Read the model definition and answer for the solid it produces. Units are mm, in the model's axes. A direction names the side the tool comes from. Coordinates: 2 decimals unless noted, no trailing zeros. Loops run counter-clockwise (first coordinate to the right, second up) from the corner with the lowest first, then second, coordinate; pieces in that order, holes last. Notation, with made-up numbers: (30, 18) - (85, 18) arc R5 cw to (85, 27) - close; hole circle Ø8 at (-9.75, -1). An arc over 180 degrees is marked (long way). Use one line per item in the form item = value. Start each with the question number.
1) A cutting plane is placed at B-B (y = 0). Give the vertices of the cut face in (x, z).
2) A cutting plane is placed at D-D (y = -41.5). Give the vertices of the cut face in (x, z), and give its area (3 significant figures).
3) Consider line 1 (X direction, y = -38, z = 11); line 2 (Y direction, x = -3, z = 69.5); line 3 (Z direction, x = 12.5, y = 15). Determine where each line is inside the solid, lowest interval first.
4) Which of the six approach directions +Z, -Z, +X, -X, +Y, -Y give full straight-line access (tool end or side, diameter ignored) to faces 1 (the face through (-16.31, -19.16, 17.93)), 2 (the face through (40.94, -29.63, 35.74)), 3 (the face through (8.89, 17, 10)), 4 (the face through (-36, -92, 11)), 5 (the face through (-1, -76.2, -46))?
5) The mould has two halves that part along Z. Classify faces 6 (the face through (37, -92, 8)), 7 (the face through (-36.437, -62.42, 9.311)), 8 (the face through (-48.89, 23.59, 10.2)), 9 (the face through (-0.4, -63.3, 32.5)): released by +Z, released by -Z, zero draft, split by the parting line, or undercut.
6) Each of these flat-tipped pins is pushed along its axis until it touches: P1, Ø4, axis at x = -15.5, y = -15.5, coming from the -Z side; P2, Ø4, axis at x = -35, y = -21, coming from the +Z side; P3, Ø1, axis at x = 7, z = 1, coming from the +Y side; P4, Ø12, axis at x = -6.5, z = 9, coming from the +Y side. Where does it stop, or does it pass through?
7) A cutting plane is placed at A-A (x = 0). Give the vertices of the cut face in (y, z).
8) A cutting plane is placed at C-C (z = 10). State how many separate pieces and enclosed holes the cut face has, and give its area (3 significant figures).
from build123d import *

# Parameters (mm, degrees)
BOSS_EXTRUDE1_DEPTH = 20
SKETCH2_R           = 16.25
SKETCH2_R_2         = 2.15
CUT_EXTRUDE1_DEPTH  = 20
SKETCH5_R           = 3.75
CUT_EXTRUDE4_DEPTH  = 4.2
FILLET3_R           = 4
SKETCH6_W           = 101.6
SKETCH6_H           = 152.4
BOSS_EXTRUDE2_DEPTH = 20
SKETCH7_R           = 3.75
CUT_EXTRUDE5_DEPTH  = 4.2
SKETCH8_R           = 1.8
CUT_EXTRUDE6_DEPTH  = 60
CHAMFER1_SIZE       = 25.4
BOSS_EXTRUDE4_DEPTH = 20
FILLET4_R           = 6.35
CUT_EXTRUDE8_DEPTH  = 165.339404891
CUT_EXTRUDE9_DEPTH  = 165.339404891


with BuildPart() as part:
    # Sketch1 → Boss-Extrude1 (new body)
    with BuildSketch(Plane.XY):
        Polygon((50.8, 25.4), (8.89, 25.4), (8.89, 13.302928249), (-8.89, 13.302928249), (-8.89, 25.4), (-50.8, 25.4), (-50.8, -76.2), (50.8, -76.2), align=None)
    extrude(amount=BOSS_EXTRUDE1_DEPTH)

    # Sketch2 → Cut-Extrude1 (cut)
    with BuildSketch(Plane.XY.offset(20)):
        Circle(SKETCH2_R)
        with Locations((-15.5, -15.5)):
            Circle(SKETCH2_R_2)
        with Locations((-15.5, 15.5)):
            Circle(SKETCH2_R_2)
        with Locations((15.5, -15.5)):
            Circle(SKETCH2_R_2)
        with Locations((15.5, 15.5)):
            Circle(SKETCH2_R_2)
    extrude(amount=-CUT_EXTRUDE1_DEPTH, mode=Mode.SUBTRACT)

    # Sketch5 → Cut-Extrude4 (cut)
    with BuildSketch(Plane.XY.offset(20)):
        with Locations((-15.5, 15.5)):
            Circle(SKETCH5_R)
        with Locations((15.5, 15.5)):
            Circle(SKETCH5_R)
        with Locations((15.5, -15.5)):
            Circle(SKETCH5_R)
        with Locations((-15.5, -15.5)):
            Circle(SKETCH5_R)
    extrude(amount=-CUT_EXTRUDE4_DEPTH, mode=Mode.SUBTRACT)

    # Fillet3
    fillet3_edges = [part.edges().sort_by_distance(p)[0] for p in [
        (8.89, 13.602587989, 10),
        (-8.89, 13.602587989, 10),
    ]]
    fillet(fillet3_edges, radius=FILLET3_R)

    # Sketch6 → Boss-Extrude2 (add)
    with BuildSketch(Plane.XZ.offset(76.2)):
        with Locations((0, 10)):
            Rectangle(SKETCH6_W, SKETCH6_H)
    extrude(amount=BOSS_EXTRUDE2_DEPTH)

    # Sketch7 → Cut-Extrude5 (cut)
    with BuildSketch(Plane.XZ.offset(96.2)):
        with Locations((-38.1, 10)):
            Circle(SKETCH7_R)
        with Locations((38.1, 10)):
            Circle(SKETCH7_R)
        with Locations((0, 10)):
            Circle(SKETCH7_R)
    extrude(amount=-CUT_EXTRUDE5_DEPTH, mode=Mode.SUBTRACT)

    # Sketch8 → Cut-Extrude6 (cut)
    with BuildSketch(Plane.XZ.offset(92)):
        with Locations((-38.1, 10)):
            Circle(SKETCH8_R)
        with Locations((38.1, 10)):
            Circle(SKETCH8_R)
        with Locations((0, 10)):
            Circle(SKETCH8_R)
    extrude(amount=-CUT_EXTRUDE6_DEPTH, mode=Mode.SUBTRACT)

    # Chamfer1
    chamfer1_edges = [part.edges().sort_by_distance(p)[0] for p in [
        (0, -76.2, 0),
        (0, -76.2, 20),
    ]]
    chamfer(chamfer1_edges, length=CHAMFER1_SIZE)

    # Sketch12 → Boss-Extrude4 (add)
    with BuildSketch(Plane(origin=(50.8, 0, 0), x_dir=(0, 0, -1), z_dir=(1, 0, 0))):
        Polygon((-86.2, -76.2), (-20, 25.4), (-20, -76.2), align=None)
        Polygon((0, -76.2), (66.2, -76.2), (0, 25.4), align=None)
    boss_extrude4 = extrude(amount=-BOSS_EXTRUDE4_DEPTH)

    # Mirror2: Boss-Extrude4 across plane
    add(boss_extrude4.mirror(Plane(origin=(0, 0, 0), x_dir=(0, 0, 1), z_dir=(1, 0, 0))))

    # Fillet4
    fillet4_edges = [part.edges().sort_by_distance(p)[0] for p in [
        (50.8, -86.2, -66.2),
        (50.8, -86.2, 86.2),
        (-50.8, -86.2, 86.2),
        (-50.8, -86.2, -66.2),
        (-50.8, 25.4, 10),
        (-8.89, 25.4, 10),
        (8.89, 25.4, 10),
        (50.8, 25.4, 10),
        (30.8, -12.7, 20),
        (30.8, -12.7, 0),
        (-30.8, -12.7, 20),
        (-30.8, -12.7, 0),
    ]]
    fillet(fillet4_edges, radius=FILLET4_R)

    # Sketch16 → Cut-Extrude8 (cut, through all)
    with BuildSketch(Plane.ZY.offset(50.8)):
        Polygon((-66.2, -76.2), (-25.4, -76.2), (-6.35, 15.654380665), align=None)
    extrude(amount=-CUT_EXTRUDE8_DEPTH, mode=Mode.SUBTRACT)

    # Sketch14 → Cut-Extrude9 (cut, through all)
    with BuildSketch(Plane(origin=(50.8, 0, 0), x_dir=(0, 0, -1), z_dir=(1, 0, 0))):
        Polygon((-86.2, -76.2), (-26.35, 15.654380665), (-45.4, -76.2), align=None)
    extrude(amount=-CUT_EXTRUDE9_DEPTH, mode=Mode.SUBTRACT)


solid = part.part
Found:
q1.outline = (-50.8, -9.6) - (-30.8, -9.6) - (-30.8, -6.35) arc R6.35 cw to (-24.45, 0) - (-16.25, 0) - (-16.25, 20) - (-24.45, 20) arc R6.35 cw to (-30.8, 26.35) - (-30.8, 29.6) - (-50.8, 29.6) - close; (16.25, 0) - (24.45, 0) arc R6.35 cw to (30.8, -6.35) - (30.8, -9.6) - (50.8, -9.6) - (50.8, 29.6) - (30.8, 29.6) - (30.8, 26.35) arc R6.35 cw to (24.45, 20) - (16.25, 20) - close
q2.outline = (-50.8, -18.2) - (-30.8, -18.2) - (-30.8, -6.35) arc R6.35 cw to (-24.45, 0) - (24.45, 0) arc R6.35 cw to (30.8, -6.35) - (30.8, -18.2) - (50.8, -18.2) - (50.8, 38.2) - (30.8, 38.2) - (30.8, 26.35) arc R6.35 cw to (24.45, 20) - (-24.45, 20) arc R6.35 cw to (-30.8, 26.35) - (-30.8, 38.2) - (-50.8, 38.2) - close; hole circle Ø3.6 at (-38.1, 10); hole circle Ø3.6 at (0, 10); hole circle Ø3.6 at (38.1, 10)
q2.area = 3,490 mm^2
q3.line_1 = -50.8 to -39.6, -36.6 to -1.5, 1.5 to 36.6, 39.6 to 50.8
q3.line_2 = -96.2 to -76.2
q3.line_3 = 0 to 15.8
q4.face_1 = +Z
q4.face_2 = +Z, +X, -X, +Y
q4.face_3 = +Z, -Z, +Y
q4.face_4 = -Y
q4.face_5 = -Z, +X, -X, +Y
q5.face_6 = undercut
q5.face_7 = undercut
q5.face_8 = zero draft
q5.face_9 = released by +Z
q6.P1 = through
q6.P2 = 34.37
q6.P3 = -14.42
q6.P4 = 24.78
q7.outline = (-96.2, -66.2) - (-76.2, -66.2) - (-76.2, -25.4) - (-50.8, 0) - (-16.25, 0) - (-16.25, 20) - (-50.8, 20) - (-76.2, 45.4) - (-76.2, 86.2) - (-96.2, 86.2) - (-96.2, 13.75) - (-92, 13.75) - (-92, 11.8) - (-32, 11.8) - (-32, 8.2) - (-92, 8.2) - (-92, 6.25) - (-96.2, 6.25) - close
q8.separate_pieces = 1
q8.enclosed_holes = 4
q8.area = 10,500 mm^2
